Model file for the job. Use its own axes, mm. A direction names the side the tool comes from. Give positions to 0.01 mm unless a question says otherwise; leave off trailing zeros. Order: outer loops, then holes, each group sorted by start corner. A loop starts at its lowest first (then second) coordinate and runs counter-clockwise, first axis right, second up. Notation, with made-up numbers: M 5,5 L 24,5 A17 cw 24,13 Z; hole C 9.25,89.5 d3. An arc over 180 degrees is marked long. Return JSON: item names as keys, results as strings. Group by question number.
1. Slice it at B-B on x = 4.5. List the corners of the cut face in (y, z).
2. Wall check: probe 1 along X at (y, z) = (16.5, -1); probe 2 along X at (y, z) = (-6, 4.25); probe 3 along Y at (x, z) = (-16, 7.5). Give the ranges that are in metal, low to high. Write a range as [from, to].
3. Slice it at C-C on z = 5.75. List the corners of the cut face in (x, y), then the cut area to 3 significant figures.
4. Pin check, flat tips, straight feed: pin 1 (1.5 mm diameter, centred on y = 34.5, z = -1.5, fed in from -X); pin 2 (2.5 mm diameter, centred on x = -2.5, z = -2, fed in from -Y). Stop position of each tip, or through.
5. Slice it at A-A on y = 0.5. List the corners of the cut face in (x, z), then the cut area to 3 significant figures.
6. Two-plate mould, pull along X, no slides. Class faces 1 (the face through (0, -45.523, 3)), 2 (the face through (0, 49.977, -1)), 3 (the face through (1, 49.477, 3)), 4 (the face through (30.322, 1, 4)): released by +X, released by -X, zero draft, split by the parting line, or undercut.
7. 3-axis set-ups, long thin cutter, end or side, ignore diameter. For faces 5 (the face through (1, -46.023, -1)), 6 (the face through (-25.272, -43.742, -1.479)), 7 (the face through (28.322, 3, -1)), 8 (the face through (-27.178, 3, 3)), 9 (the face through (26.04, -43.62, -1.48)): which of +Z, -Z, +X, -X, +Y, -Y reach the whole face in a straight line?
from build123d import *

# Parameters (mm, degrees)
F0_W     = 60
F0_H     = 100
F1_DEPTH = 12
F2_R     = 10
F3_R     = 3
F4_T     = -2.5
F6_DEPTH = 3


with BuildPart() as f1:
    # F0 (on Top) → F1 (new body)
    with BuildSketch(Plane.XY):
        with Locations((0.322031, 1.976583)):
            Rectangle(F0_W, F0_H)
    extrude(amount=F1_DEPTH)

    # F2
    f2_edges = [f1.edges().sort_by_distance(p)[0] for p in [
        (-29.677969, -48.023417, 6),
        (-29.677969, 51.976583, 6),
        (30.322031, -48.023417, 6),
        (30.322031, 51.976583, 6),
    ]]
    fillet(f2_edges, radius=F2_R)

    # F3
    f3_edges = [f1.edges().sort_by_distance(p)[0] for p in [
        (0.322031, 51.976583, 12),
    ]]
    fillet(f3_edges, radius=F3_R)

    # F4
    f4_openings = [f1.faces().sort_by_distance(p)[0] for p in [
        (0.322031, 1.976583, 0),
    ]]
    offset(amount=F4_T, openings=f4_openings)

    # F5 (on face) → F6 (join)
    with BuildSketch(Plane(origin=(0, 0, 0), x_dir=(1, 0, 0), z_dir=(0, 0, -1))):
        with BuildLine():
            Line((-27.677969, 38.023417), (-27.677969, -41.976583))
            ThreePointArc((-27.677969, -41.976583), (-25.334823, -47.633437), (-19.677969, -49.976583))
            Line((-19.677969, -49.976583), (20.322031, -49.976583))
            ThreePointArc((20.322031, -49.976583), (25.978885, -47.633437), (28.322031, -41.976583))
            Line((28.322031, -41.976583), (28.322031, 38.023417))
            ThreePointArc((28.322031, 38.023417), (25.978885, 43.680271), (20.322031, 46.023417))
            Line((20.322031, 46.023417), (-19.677969, 46.023417))
            ThreePointArc((-19.677969, 46.023417), (-25.334823, 43.680271), (-27.677969, 38.023417))
        make_face()
        with BuildLine():
            ThreePointArc((-19.677969, -49.476583), (-24.98127, -47.279884), (-27.177969, -41.976583))
            Line((-27.177969, -41.976583), (-27.177969, 38.023417))
            ThreePointArc((-27.177969, 38.023417), (-24.98127, 43.326718), (-19.677969, 45.523417))
            Line((-19.677969, 45.523417), (20.322031, 45.523417))
            ThreePointArc((20.322031, 45.523417), (25.625332, 43.326718), (27.822031, 38.023417))
            Line((27.822031, 38.023417), (27.822031, -41.976583))
            ThreePointArc((27.822031, -41.976583), (25.625332, -47.279884), (20.322031, -49.476583))
            Line((20.322031, -49.476583), (-19.677969, -49.476583))
        make_face(mode=Mode.SUBTRACT)
    extrude(amount=F6_DEPTH)


solid = f1.part
Result:
{
 "1": {"outline": "M -48.02,0 L -46.02,0 L -46.02,-3 L -45.52,-3 L -45.52,9 A0.5 cw -45.02,9.5 L 48.98,9.5 A0.5 cw 49.48,9 L 49.48,-3 L 49.98,-3 L 49.98,0 L 51.98,0 L 51.98,9 A3 ccw 48.98,12 L -45.02,12 A3 ccw -48.02,9 Z"},
 "2": {"probe 1": "x = [-27.68, -27.18], [27.82, 28.32]", "probe 2": "x = [-29.68, -27.18], [27.82, 30.32]", "probe 3": "y = [-48.02, -45.52], [49.48, 51.98]"},
 "3": {"outline": "M -29.68,-38.02 A10 ccw -19.68,-48.02 L 20.32,-48.02 A10 ccw 30.32,-38.02 L 30.32,41.98 A10 ccw 20.32,51.98 L -19.68,51.98 A10 ccw -29.68,41.98 Z; hole M -27.18,-38.02 A7.5 ccw -19.68,-45.52 L 20.32,-45.52 A7.5 ccw 27.82,-38.02 L 27.82,41.98 A7.5 ccw 20.32,49.48 L -19.68,49.48 A7.5 ccw -27.18,41.98 Z", "area": "737 mm2"},
 "4": {"pin 1": "stops at x = -27.68", "pin 2": "stops at y = -46.02"},
 "5": {"outline": "M -29.68,0 L -27.68,0 L -27.68,-3 L -27.18,-3 L -27.18,9 A0.5 cw -26.68,9.5 L 27.32,9.5 A0.5 cw 27.82,9 L 27.82,-3 L 28.32,-3 L 28.32,0 L 30.32,0 L 30.32,9 A3 ccw 27.32,12 L -26.68,12 A3 ccw -29.68,9 Z", "area": "197 mm2"},
 "6": {"face 1": "undercut", "face 2": "zero draft", "face 3": "undercut", "face 4": "released by +X"},
 "7": {"face 5": "-Z, +X, -X, -Y", "face 6": "-Z, -X, -Y", "face 7": "-Z, +X, +Y, -Y", "face 8": "-Z", "face 9": "-Z, +X, -Y"}
}
